Check sheet for the modelled part. Datum: model origin and axes. Units: mm. Face numbers are marked on the shaded views. Give positions to 0.01 mm unless a question says otherwise; leave off trailing zeros. Write each loop counter-clockwise with the first axis right and the second up, starting at its lowest first coordinate (ties: lowest second). Pieces come first, ordered by that corner, then holes. Notation, with made-up numbers: M 59,38.25 L 75,38.25 A14 cw 75,42.25 Z; hole C 88,-1.5 d3. An arc over 180 degrees is marked long. Use CSV: the item, a comma, the result in double quotes. Start each with the question number.
1. Mould release check, pull along X, two halves, no side actions. Record for the marked faces 1 and 2: +X half, -X half, draft (parallel to the pull), parting line (faces both ways), or undercut.
2. Scan lines: line 1 (X direction, y = 2, z = -22.5); line 2 (Z direction, x = -27.5, y = 5); line 3 (Z direction, x = -12, y = 13.5). Record each from-to range of solid material in increasing order.
3. Depth check by flat-ended pin: P1, Ø10, axis at x = -10.5, z = -18, coming from the +Y side; P2, Ø12, axis at y = 9.5, z = -12, coming from the +X side; P3, Ø9.5, axis at x = 14, y = 12.5, coming from the +Z side; P4, Ø5, axis at x = 13.5, z = -11, coming from the +Y side. Enter the tip coordinate at first touch or a pass-through.
4. Cross-section at A-A, the plane x = -1.5. Enter the section's corners in (y, z), and give its area (3 significant figures).
from build123d import *

# Parameters (mm, degrees)
SHELL1_T = -1


with BuildPart() as part:
    # Sketch1 → Loft2 section 0
    with BuildSketch(Plane(origin=(0, 0, 0), x_dir=(1, 0, 0), z_dir=(0, 1, 0))):
        with BuildLine():
            Line((-31.199529688, 24.851146384), (30.800470312, 24.851146384))
            Line((30.800470312, 24.851146384), (30.800470312, 4.851146384))
            Line((30.800470312, 4.851146384), (-31.199529688, 4.851146384))
            Line((-31.199529688, 4.851146384), (-31.199529688, 24.851146384))
        make_face()
    # Sketch2 → Loft2 section 1
    with BuildSketch(Plane(origin=(0, 20, 0), x_dir=(1, 0, 0), z_dir=(0, 1, 0))):
        with BuildLine():
            Line((-31.199529688, 24.851146384), (30.800470312, 24.851146384))
            Line((30.800470312, 24.851146384), (30.800470312, 23.851146384))
            Line((30.800470312, 23.851146384), (-31.199529688, 23.851146384))
            Line((-31.199529688, 23.851146384), (-31.199529688, 24.851146384))
        make_face()
    loft()

    # Shell1
    shell1_openings = [part.faces().sort_by_distance(p)[0] for p in [
        (-0.199529688, 0, -14.851146384),
    ]]
    offset(amount=SHELL1_T, openings=shell1_openings, kind=Kind.INTERSECTION)


solid = part.part
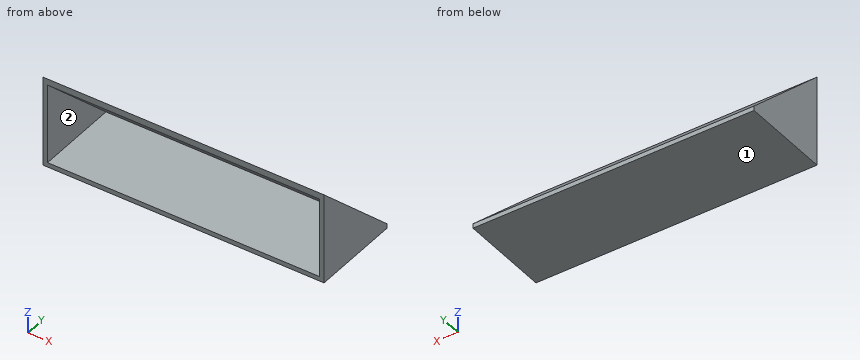
Worked answers:
1,face 1,"draft"
1,face 2,"undercut"
2,line 1,"x = -31.2 to -30.2, 29.8 to 30.8"
2,line 2,"z = -24.85 to -23.85, -10.98 to -9.6"
2,line 3,"z = -24.85 to -23.85, -19.06 to -17.68"
3,P1,"stops at y = 19.1"
3,P2,"stops at x = 30.8"
3,P3,"stops at z = -12.21"
3,P4,"stops at y = 9.1"
4,outline,"M 0,-24.85 L 20,-24.85 L 20,-23.85 L 0,-4.85 L 0,-6.23 L 18.55,-23.85 L 0,-23.85 Z"
4,area,"46.6 mm^2"
